```python
from build123d import *

# Parameters (mm, degrees)
SKETCH1_W           = 111.76
SKETCH1_H           = 19.05
BOSS_EXTRUDE1_DEPTH = 5.08
SKETCH5_W           = 5.08
SKETCH5_H           = 5.08
BOSS_EXTRUDE3_DEPTH = 12.7
FILLET2_R           = 7.62
SKETCH7_W           = 5.08
SKETCH7_H           = 12.7
CUT_EXTRUDE2_DEPTH  = 61.35173092


with BuildPart() as part:
    # Sketch1 → Boss-Extrude1 (new body)
    with BuildSketch(Plane.XY):
        Rectangle(SKETCH1_W, SKETCH1_H)
    extrude(amount=BOSS_EXTRUDE1_DEPTH)

    # Sketch5 → Boss-Extrude3 (add)
    with BuildSketch(Plane.XZ.offset(9.525)):
        with Locations((-53.34, 2.54)):
            Rectangle(SKETCH5_W, SKETCH5_H)
    boss_extrude3 = extrude(amount=BOSS_EXTRUDE3_DEPTH)

    # Mirror1: Boss-Extrude3 across plane
    add(boss_extrude3.mirror(Plane(origin=(0, 0, 0), x_dir=(0, 0, 1), z_dir=(1, 0, 0))))

    # Fillet2
    # the kernel refuses this fillet: 7.62 mm, written as the material it takes off along each edge
    with BuildSketch(Plane(origin=(-55.88, -22.225, -17.960512242), x_dir=(1, 0, 0), z_dir=(0, 0, 1))) as fillet2_piece_1:
        with BuildLine():
            CenterArc((7.62, 7.184204897), FILLET2_R, 180, 70.528779366)
            Line((0, 7.184204897), (-0.1524, 7.184204897))
            Line((-0.1524, 7.184204897), (-0.1524, 0))
            Line((-0.1524, 0), (0, -0.1524))
            ThreePointArc((0, -0.1524), (2.54, -0.1524), (5.0292, -0.143684098))
            Line((5.0292, -0.143684098), (5.08, 0))
        make_face()
    extrude(amount=41.001024484, mode=Mode.SUBTRACT)
    with BuildSketch(Plane(origin=(55.88, -22.225, -17.960512242), x_dir=(0, 1, 0), z_dir=(0, 0, 1))) as fillet2_piece_2:
        with BuildLine():
            CenterArc((7.184204897, 7.62), FILLET2_R, 199.471220634, 70.528779366)
            Line((0, 5.08), (-0.143684098, 5.0292))
            ThreePointArc((-0.143684098, 5.0292), (-0.1524, 2.54), (-0.1524, 0))
            Line((-0.1524, 0), (0, -0.1524))
            Line((0, -0.1524), (7.184204897, -0.1524))
            Line((7.184204897, -0.1524), (7.184204897, 0))
        make_face()
    extrude(amount=41.001024484, mode=Mode.SUBTRACT)

    # Sketch7 → Cut-Extrude2 (cut, through all)
    with BuildSketch(Plane.XY.offset(5.08)):
        with Locations((0, 3.175)):
            Rectangle(SKETCH7_W, SKETCH7_H)
    extrude(amount=-CUT_EXTRUDE2_DEPTH, mode=Mode.SUBTRACT)


solid = part.part
```
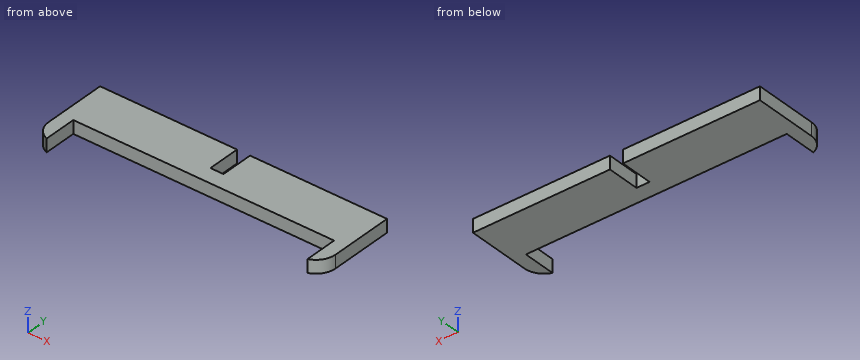
CAD build for the part. Positions are in the model's coordinates, mm. Round coordinates to 2 decimals unless told otherwise and drop trailing zeros. Order: outer loops, then holes, each group sorted by start corner. A loop starts at its lowest first (then second) coordinate and runs counter-clockwise, first axis right, second up.
Q1. Slice it at A-A (y = 6). Write the cut outline in (x, z).
Q2. Wall check: L1, parallel to X at y = -13, z = 2.2; L2, parallel to X at y = 3, z = 4.2; L3, parallel to Y at x = 32, z = 1.65 (3 decimals). Give the ranges that are in metal, low to high.
Q3. Drop flat-ended pins along their axis: pin 1 (2.5 mm diameter, centred on x = 0, z = 2.5, fed in from -Y) (3 decimals); pin 2 (2 mm diameter, centred on y = -16.5, z = 4, fed in from -X). Give the stop position or say it passes through.
Q4. Slice it at C-C (y = -13.5). Write the cut outline in (x, z).
Q5. Slice it at B-B (z = 1.95). Write the cut outline in (x, y) (3 decimals).
Q6. Slice it at D-D (x = 42). Write the cut outline in (y, z) (3 decimals), and give its area (3 significant figures).
Results below:
1. outline: (-55.88, 0) - (-2.54, 0) - (-2.54, 5.08) - (-55.88, 5.08) - close; (2.54, 0) - (55.88, 0) - (55.88, 5.08) - (2.54, 5.08) - close
2. L1: x = -55.88 to -50.8, 50.8 to 55.88
2. L2: x = -55.88 to -2.54, 2.54 to 55.88
2. L3: y = -9.525 to 9.525
3. pin 1: stops at y = -9.525
3. pin 2: stops at x = -55.87
4. outline: (-55.88, 0) - (-50.8, 0) - (-50.8, 5.08) - (-55.88, 5.08) - close; (50.8, 0) - (55.88, 0) - (55.88, 5.08) - (50.8, 5.08) - close
5. outline: (-55.88, -15.041) arc R7.62 ccw to (-50.8, -22.225) - (-50.8, -9.525) - (50.8, -9.525) - (50.8, -22.225) arc R7.62 ccw to (55.88, -15.041) - (55.88, 9.525) - (2.54, 9.525) - (2.54, -3.175) - (-2.54, -3.175) - (-2.54, 9.525) - (-55.88, 9.525) - close
6. outline: (-9.525, 0) - (9.525, 0) - (9.525, 5.08) - (-9.525, 5.08) - close
6. area: 96.8 mm2
